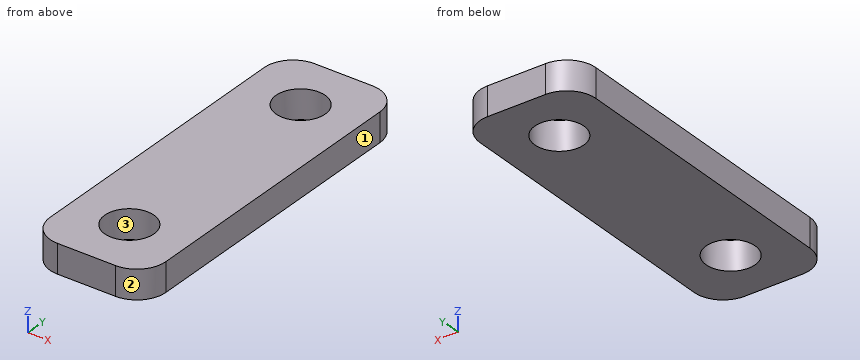
```python
from build123d import *

# Parameters (mm, degrees)
ESQUISSE1_W             = 40
ESQUISSE1_H             = 120
BOSS_EXTRU_1_DEPTH      = 5
ESQUISSE2_R             = 8.5
ENL_V_MAT_EXTRU_1_DEPTH = 11
CONG_1_R                = 10


with BuildPart() as part:
    # Esquisse1 → Boss.-Extru.1 (new body, symmetric)
    with BuildSketch(Plane.XY):
        with Locations((70, 0)):
            Rectangle(ESQUISSE1_W, ESQUISSE1_H)
    extrude(amount=BOSS_EXTRU_1_DEPTH, both=True)

    # Esquisse2 → Enlèv. mat.-Extru.1 (cut, through all)
    with BuildSketch(Plane.XY.offset(5)):
        with Locations((70, 40)):
            Circle(ESQUISSE2_R)
        with Locations((70, -40)):
            Circle(ESQUISSE2_R)
    extrude(amount=-ENL_V_MAT_EXTRU_1_DEPTH, mode=Mode.SUBTRACT)

    # Congé1
    cong_1_edges = [part.edges().sort_by_distance(p)[0] for p in [
        (50, 60, 0),
        (90, 60, 0),
        (90, -60, 0),
        (50, -60, 0),
    ]]
    fillet(cong_1_edges, radius=CONG_1_R)


solid = part.part
```
Work out the finished part from the listing and answer in its coordinate system (mm). Face numbers are marked on the shaded views. Round coordinates to 2 decimals unless told otherwise and drop trailing zeros. Loops run counter-clockwise (first coordinate to the right, second up) from the corner with the lowest first, then second, coordinate; pieces in that order, holes last.
(1) Find the intervals of material crossed by L1, parallel to Y at x = 70, z = -0.5; L2, parallel to Y at x = 67, z = 1; L3, parallel to X at y = -45.5, z = -3.25, in increasing order.
Computed values:
L1: y = -60 to -48.5, -31.5 to 31.5, 48.5 to 60
L2: y = -60 to -47.95, -32.05 to 32.05, 47.95 to 60
L3: x = 50 to 63.52, 76.48 to 90
(2) The part is cut by section B-B, the plane z = -3. Give the vertices of the cut face in (x, y), and give its area (3 significant figures).
Computed values:
outline: (50, -50) arc R10 ccw to (60, -60) - (80, -60) arc R10 ccw to (90, -50) - (90, 50) arc R10 ccw to (80, 60) - (60, 60) arc R10 ccw to (50, 50) - close; hole circle Ø17 at (70, -40); hole circle Ø17 at (70, 40)
area: 4,260 mm2
(3) The part is cut by section D-D, the plane x = 55. Give the vertices of the cut face in (y, z), and give its area (3 significant figures).
Computed values:
outline: (-58.66, -5) - (58.66, -5) - (58.66, 5) - (-58.66, 5) - close
area: 1,170 mm2
(4) Each of these flat-tipped pins is pushed along its axis until it touches: P1, Ø1.5, axis at x = 56.5, z = 1.5, coming from the +Y side; P2, Ø22, axis at x = 70, y = 40, coming from the -Z side; P3, Ø13.5, axis at x = 70, y = -40, coming from the -Z side. Where does it stop, or does it pass through?
Computed values:
P1: stops at y = 59.61
P2: stops at z = -5
P3: passes through
(5) The part is cut by section C-C, the plane x = 70. Give the vertices of the cut face in (y, z), and give its area (3 significant figures).
Computed values:
outline: (-60, -5) - (-48.5, -5) - (-48.5, 5) - (-60, 5) - close; (-31.5, -5) - (31.5, -5) - (31.5, 5) - (-31.5, 5) - close; (48.5, -5) - (60, -5) - (60, 5) - (48.5, 5) - close
area: 860 mm2
(6) The part is cut by section A-A, the plane y = -40. Give the vertices of the cut face in (x, z).
Computed values:
outline: (50, -5) - (61.5, -5) - (61.5, 5) - (50, 5) - close; (78.5, -5) - (90, -5) - (90, 5) - (78.5, 5) - close
(7) The mould has two halves that part along Y. Classify the marked faces 1, 2 and 3: pulls with the +Y half, pulls with the -Y half, needs draft (parallel to the pull), parting line crosses it, or undercut.
Computed values:
face 1: needs draft
face 2: pulls with the -Y half
face 3: undercut
